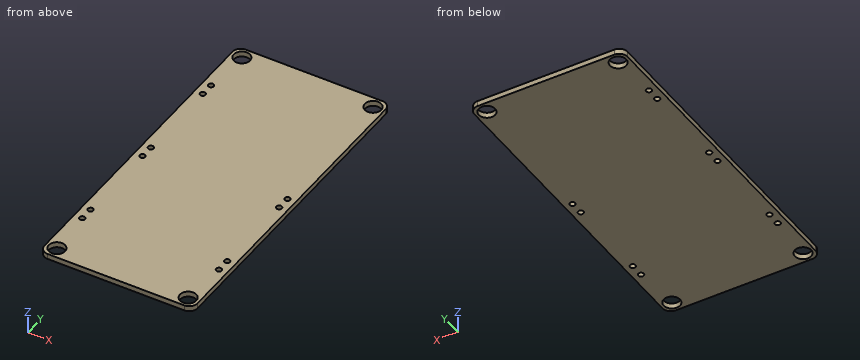
```python
from build123d import *

# Parameters (mm, degrees)
SKETCH_R     = 1.5
PAD_DEPTH    = 1
SKETCH001_R  = 0.5
POCKET_DEPTH = 1.001


with BuildPart() as part:
    # Sketch → Pad (new body)
    with BuildSketch(Plane.XY):
        with BuildLine():
            Line((-12.5, 30), (12.5, 30))
            ThreePointArc((14, 28.5), (13.56066, 29.56066), (12.5, 30))
            Line((14, 28.5), (14, -28.5))
            ThreePointArc((12.5, -30), (13.56066, -29.56066), (14, -28.5))
            Line((12.5, -30), (-12.5, -30))
            ThreePointArc((-14, -28.5), (-13.56066, -29.56066), (-12.5, -30))
            Line((-14, -28.5), (-14, 28.5))
            ThreePointArc((-12.5, 30), (-13.56066, 29.56066), (-14, 28.5))
        make_face()
        with Locations((-12, 28)):
            Circle(SKETCH_R, mode=Mode.SUBTRACT)
        with Locations((12, 28)):
            Circle(SKETCH_R, mode=Mode.SUBTRACT)
        with Locations((-12, -28)):
            Circle(SKETCH_R, mode=Mode.SUBTRACT)
        with Locations((12, -28)):
            Circle(SKETCH_R, mode=Mode.SUBTRACT)
    extrude(amount=PAD_DEPTH)

    # Sketch001 → Pocket (cut, through all)
    with BuildSketch(Plane.XY):
        with Locations((-12.5, 19.5)):
            Circle(SKETCH001_R)
        with Locations((-12.5, 17)):
            Circle(SKETCH001_R)
        with Locations((-12.5, 1.25)):
            Circle(SKETCH001_R)
        with Locations((-12.5, -1.25)):
            Circle(SKETCH001_R)
        with Locations((-12.5, -17)):
            Circle(SKETCH001_R)
        with Locations((-12.5, -19.5)):
            Circle(SKETCH001_R)
        with Locations((12.5, -17)):
            Circle(SKETCH001_R)
        with Locations((12.5, -19.5)):
            Circle(SKETCH001_R)
        with Locations((12.5, 1.25)):
            Circle(SKETCH001_R)
        with Locations((12.5, -1.25)):
            Circle(SKETCH001_R)
    extrude(amount=POCKET_DEPTH, mode=Mode.SUBTRACT)


solid = part.part
```
Source: CAD feature listing. Evaluate the final solid. Frame: model axes, mm. Give positions to 0.01 mm unless a question says otherwise; leave off trailing zeros. Put each result on its own line as item: value.
Q1. Pin query (flat end, axial travel): P1, Ø2.5, axis at x = -12, y = 28, coming from the -Z side. Return the tip coordinate at first contact, or that it passes through.
Response values:
P1: passes through
Q2. Section A-A (z = 0.6). Count the separate pieces of the cut face and the enclosed holes in it, and give its area (3 significant figures).
Response values:
separate pieces: 1
enclosed holes: 14
area: 1,640 mm²
Q3. Line query: probe 1 along X at (y, z) = (-17, 0.55); probe 2 along Y at (x, z) = (-11.75, 0.8); probe 3 along X at (y, z) = (-1, 0.45). Output: solid intervals per line, ascending. Write a range as [from, to].
Response values:
probe 1: x = [-14, -13], [-12, 12], [13, 14]
probe 2: y = [-30, -29.48], [-26.52, 26.52], [29.48, 30]
probe 3: x = [-14, -12.93], [-12.07, 12.07], [12.93, 14]
